Can you work these out from the drawing? Everything is in mm from the part's minimum corner. A direction names the side the tool comes from. Round coordinates to 2 decimals unless told otherwise and drop trailing zeros. Write each loop counter-clockwise with the first axis right and the second up, starting at its lowest first coordinate (ties: lowest second). Pieces come first, ordered by that corner, then holes. Notation, with made-up numbers: M -0.5,77.5 L 41.5,77.5 A28 ccw 41.5,95.5 Z; hole C -38.75,-31 d4. An arc over 180 degrees is marked long. Use one line per item in the form item = value. Start each with the question number.
Q1. I want a section at B-B on y = 2.5. List the corners of the cut face in (x, z) for me.
Q2. I need wall thicknesses on line 1 along Y through (x, z) = (19, 4.5); line 2 along X through (y, z) = (4.5, 8); line 3 along Y through (x, z) = (6.5, 5.75). Which ranges of each line are inside material? Lowest first, please. Write a range as from..to.
Q3. We'd pull the mould along X, two halves only. Please class the marked faces 1, 2, 3 and 4: +X half, -X half, draft (parallel to the pull), parting line (faces both ways), or undercut.
Q4. I want a section at A-A on x = 19. List the corners of the cut face in (y, z) for me.
Q5. For the marked faces 5, 6, 7 and 8, which set-ups out of +Z, -Z, +X, -X, +Y, -Y let a thin tool reach every point of the face, with its end or its side?
Q6. I want a section at C-C on z = 0.75. List the corners of the cut face in (x, y) for me, and give its area (3 significant figures).
Q7. I'm going to push flat-ended pins straight in: pin 1 Ø4 at (x, z) = (27.5, 8.5) entering from +Y; pin 2 Ø5 at (x, z) = (24, 7) entering from +Y; pin 3 Ø2.5 at (x, z) = (4, 3.5) entering from +Y. Where does each tip first touch, or does it pass through?
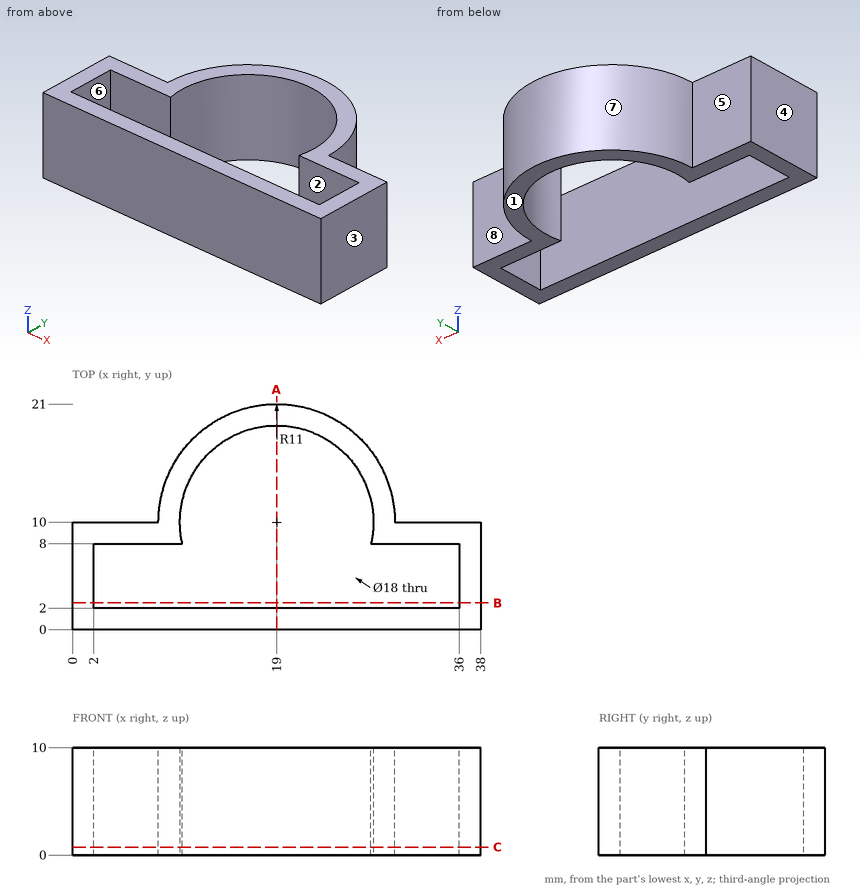
Reported:
q1.outline = M 0,0 L 2,0 L 2,10 L 0,10 Z; M 36,0 L 38,0 L 38,10 L 36,10 Z
q2.line_1 = 0..2, 19..21
q2.line_2 = 0..2, 36..38
q2.line_3 = 0..2, 8..10
q3.face_1 = draft
q3.face_2 = undercut
q3.face_3 = +X half
q3.face_4 = -X half
q4.outline = M 0,0 L 2,0 L 2,10 L 0,10 Z; M 19,0 L 21,0 L 21,10 L 19,10 Z
q5.face_5 = +Z, -Z, -X, +Y
q5.face_6 = +Z, -Z
q5.face_7 = +Z, -Z, +Y
q5.face_8 = +Z, -Z, +X, +Y
q6.outline = M 0,0 L 38,0 L 38,10 L 30,10 A11 ccw 8,10 L 0,10 Z; hole M 2,2 L 36,2 L 36,8 L 27.77,8 A9 ccw long 10.23,8 L 2,8 Z
q6.area = 203 mm^2
q7.pin_1 = 18.87
q7.pin_2 = 20.71
q7.pin_3 = 10
